Read the model definition and answer for the solid it produces. Units are mm, in the model's axes. A direction names the side the tool comes from. Coordinates: 2 decimals unless noted, no trailing zeros. Write each loop counter-clockwise with the first axis right and the second up, starting at its lowest first coordinate (ties: lowest second). Pieces come first, ordered by that corner, then holes.
from build123d import *

# Parameters (mm, degrees)
BOSS_EXTRUDE2_START   = 100
SKETCH2_R             = 75
SKETCH2_R_2           = 38
BOSS_EXTRUDE2_DEPTH   = 53
BOSS_EXTRUDE2_2_DEPTH = 53
BOSS_EXTRUDE3_START   = 106
BOSS_EXTRUDE3_DEPTH   = 41
SKETCH2_6_R           = 75
SKETCH2_6_R_2         = 38
BOSS_EXTRUDE4_DEPTH   = 100


with BuildPart() as part:
    # Sketch2 → Boss-Extrude2 (new body)
    with BuildSketch(Plane(origin=(0, 0, 0), x_dir=(0, 0, -1), z_dir=(1, 0, 0)).offset(BOSS_EXTRUDE2_START)):
        Circle(SKETCH2_R)
        Circle(SKETCH2_R_2, mode=Mode.SUBTRACT)
    boss_extrude2 = extrude(amount=BOSS_EXTRUDE2_DEPTH)



with BuildPart() as body_2:
    # Sketch2 → Boss-Extrude2 2 (new body)
    with BuildSketch(Plane(origin=(0, 0, 0), x_dir=(0, 0, -1), z_dir=(1, 0, 0)).offset(BOSS_EXTRUDE2_START)):
        with Locations((460, 0)):
            Circle(SKETCH2_R)
        with Locations((460, 0)):
            Circle(SKETCH2_R_2, mode=Mode.SUBTRACT)
    boss_extrude2_2 = extrude(amount=BOSS_EXTRUDE2_2_DEPTH)


with BuildPart() as part_1:
    add(part.part)

    add(body_2.part)  # Boss-Extrude3 merges body 2
    # Sketch2<5> → Boss-Extrude3 (add)
    with BuildSketch(Plane(origin=(0, 0, 0), x_dir=(0, 0, -1), z_dir=(1, 0, 0)).offset(BOSS_EXTRUDE3_START)):
        with BuildLine():
            ThreePointArc((0, 75), (53.033008589, 53.033008589), (75, 0))
            Line((75, 0), (385, 0))
            ThreePointArc((385, 0), (406.966991411, 53.033008589), (460, 75))
            Line((460, 75), (0, 75))
        make_face()
        with BuildLine():
            Line((385, 0), (75, 0))
            ThreePointArc((75, 0), (53.033008589, -53.033008589), (0, -75))
            Line((0, -75), (460, -75))
            ThreePointArc((460, -75), (406.966991411, -53.033008589), (385, 0))
        make_face()
    boss_extrude3 = extrude(amount=BOSS_EXTRUDE3_DEPTH)

    # Sketch2<6> → Boss-Extrude4 (add)
    with BuildSketch(Plane(origin=(0, 0, 0), x_dir=(0, 0, -1), z_dir=(1, 0, 0))):
        with Locations((460, 0)):
            Circle(SKETCH2_6_R)
        with Locations((460, 0)):
            Circle(SKETCH2_6_R_2, mode=Mode.SUBTRACT)
    boss_extrude4 = extrude(amount=BOSS_EXTRUDE4_DEPTH)

    # Mirror1: Boss-Extrude2, Boss-Extrude2 2, Boss-Extrude3, Boss-Extrude4 across plane
    add(boss_extrude2.mirror(Plane(origin=(0, 0, 0), x_dir=(0, 0, 1), z_dir=(1, 0, 0))))
    add(boss_extrude2_2.mirror(Plane(origin=(0, 0, 0), x_dir=(0, 0, 1), z_dir=(1, 0, 0))))
    add(boss_extrude3.mirror(Plane(origin=(0, 0, 0), x_dir=(0, 0, 1), z_dir=(1, 0, 0))))
    add(boss_extrude4.mirror(Plane(origin=(0, 0, 0), x_dir=(0, 0, 1), z_dir=(1, 0, 0))))


solid = part_1.part
Item 1: The part is cut by section A-A (y = 0). State how many separate pieces and enclosed holes the cut face has, and give its area (3 significant figures).
Item 2: The part is cut by section D-D (z = -484). Give the vertices of the cut face in (x, y), and give its area (3 significant figures).
Item 3: For faces 1 (the flat face through (-153, 18, -426)), 2 (the flat face through (-100, 18, 34)), 3 (the cylindrical face through (2.14, -28.73, -529.28)), determine the directions among +Z, -Z, +X, -X, +Y, -Y from which every point of the face is accessible in a straight line to the end or side of a thin tool.
Item 4: The part is cut by section C-C (x = -133). Give the vertices of the cut face in (y, z).
Item 5: Find the intervals of material crossed by probe 1 along X at (y, z) = (57.5, 19); probe 2 along X at (y, z) = (66.5, -226.5); probe 3 along Y at (x, z) = (73, -460), in increasing order.
Item 6: The part is cut by section B-B (z = -129). Give the vertices of the cut face in (x, y), and give its area (3 significant figures).
Item 7: Given pin 1 (1 mm diameter, centred on x = -41.5, y = -12.5, fed in from -Z); pin 2 (2 mm diameter, centred on x = -39, y = 38.5, fed in from +Z); pin 3 (4 mm diameter, centred on x = -12, y = -33, fed in from +Z), each flat-ended and moving along its own axis, determine where each tip first touches the part or whether it passes through.
Item 8: Determine the mould class of faces 4 (the cylindrical face through (126.129, 3.298, 74.927)), 5 (the flat face through (153, 18, -426)), 6 (the cylindrical face through (126.129, -33.713, -17.535)) for opening direction Y: +Y half, -Y half, draft (parallel to the pull), parting line (faces both ways), or undercut.
Answer:
1. separate pieces: 4
1. enclosed holes: 0
1. area: 55,900 mm2
2. outline: (-153, -71.06) - (153, -71.06) - (153, -29.46) - (-153, -29.46) - close; (-153, 29.46) - (153, 29.46) - (153, 71.06) - (-153, 71.06) - close
2. area: 25,500 mm2
3. face 1: +Z, -Z, -X, +Y, -Y
3. face 2: +Z, +Y, -Y
3. face 3: none
4. outline: (-75, -460) arc R75 ccw to (75, -460) - (75, 0) arc R75 ccw to (-75, 0) - close; hole circle Ø76 at (0, -460); hole circle Ø76 at (0, 0)
5. probe 1: x = -153 to -100, 100 to 153
5. probe 2: x = -147 to -106, 106 to 147
5. probe 3: y = -75 to -38, 38 to 75
6. outline: (-147, -75) - (-106, -75) - (-106, 75) - (-147, 75) - close; (106, -75) - (147, -75) - (147, 75) - (106, 75) - close
6. area: 12,300 mm2
7. pin 1: stops at z = -534.03
7. pin 2: stops at z = -395.05
7. pin 3: stops at z = -391.71
8. face 4: parting line
8. face 5: draft
8. face 6: undercut
